Build history of the part. All positions in model axes, mm. A direction names the side the tool comes from. Give positions to 0.01 mm unless a question says otherwise; leave off trailing zeros. Order: outer loops, then holes, each group sorted by start corner. A loop starts at its lowest first (then second) coordinate and runs counter-clockwise, first axis right, second up. Notation, with made-up numbers: (22.25, 9.5) - (29.25, 9.5) arc R6 cw to (29.25, 14.5) - close; hole circle Ø3 at (84.25, -36). An arc over 180 degrees is marked (long way). Use a Markdown table: item, result.
from build123d import *

# Parameters (mm, degrees)
SKETCH_1_R      = 1.5
SKETCH_1_R_2    = 15
EXTRUDE_1_DEPTH = 1.5


with BuildPart() as part:
    # 草圖1 → 填料-伸長1 (new body)
    with BuildSketch(Plane(origin=(0, 0, 0), x_dir=(1, 0, 0), z_dir=(0, 1, 0))):
        with BuildLine():
            Line((0, -3.980931511), (12.319060855, 2.328849967))
            ThreePointArc((12.319060855, 2.328849967), (14.431141465, 4.388450613), (15.014493405, 7.28025625))
            ThreePointArc((15.014493405, 7.28025625), (11.971039141, 65.394509034), (14.52184689, 123.53246884))
            ThreePointArc((14.52184689, 123.53246884), (15.377876917, 128.098069479), (17.067022361, 132.425226083))
            ThreePointArc((17.067022361, 132.425226083), (16.965589985, 149.77375384), (2.866920195, 159.883611111))
            ThreePointArc((2.866920195, 159.883611111), (0, 162), (-2.866920195, 159.883611111))
            ThreePointArc((-2.866920195, 159.883611111), (-16.965589985, 149.77375384), (-17.067022361, 132.425226083))
            ThreePointArc((-17.067022361, 132.425226083), (-15.377876917, 128.098069479), (-14.52184689, 123.53246884))
            ThreePointArc((-14.52184689, 123.53246884), (-11.971039141, 65.394509034), (-15.014493405, 7.28025625))
            ThreePointArc((-15.014493405, 7.28025625), (-14.431141465, 4.388450613), (-12.319060855, 2.328849967))
            Line((-12.319060855, 2.328849967), (0, -3.980931511))
        make_face()
        with Locations(Location((-12, 127.583592135, 0), (0, 0, 270))):
            Circle(SKETCH_1_R, mode=Mode.SUBTRACT)
        with Locations(Location((12, 127.583592135, 0), (0, 0, 270))):
            Circle(SKETCH_1_R, mode=Mode.SUBTRACT)
        with Locations(Location((8.6, 68.325395665, 0), (0, 0, 270))):
            Circle(SKETCH_1_R, mode=Mode.SUBTRACT)
        with Locations(Location((-8.6, 68.325395665, 0), (0, 0, 270))):
            Circle(SKETCH_1_R, mode=Mode.SUBTRACT)
        with Locations(Location((10.05, 6, 0), (0, 0, 270))):
            Circle(SKETCH_1_R, mode=Mode.SUBTRACT)
        with Locations(Location((-10.05, 6, 0), (0, 0, 270))):
            Circle(SKETCH_1_R, mode=Mode.SUBTRACT)
        with Locations(Location((0, 159, 0), (0, 0, 270))):
            Circle(SKETCH_1_R, mode=Mode.SUBTRACT)
        with Locations(Location((0, 0, 0), (0, 0, 270))):
            Circle(SKETCH_1_R, mode=Mode.SUBTRACT)
        with Locations(Location((0, 141, 0), (0, 0, 270))):
            Circle(SKETCH_1_R_2, mode=Mode.SUBTRACT)
        Polygon((0, 14.042409585), (-4.491071946, 11.449487988), (-5.101164168, 5.002829556), (5.101164168, 5.002829556), (4.491071946, 11.449487988), align=None, mode=Mode.SUBTRACT)
        with BuildLine():
            Line((0, 112.532142135), (-6.334048162, 108.875177723))
            ThreePointArc((-6.334048162, 108.875177723), (-6.614696141, 112.870067669), (-6.92146425, 116.863036776))
            Line((-6.92146425, 116.863036776), (-0.136378432, 120.780407899))
            ThreePointArc((-0.136378432, 120.780407899), (0, 120.816950389), (0.136378432, 120.780407899))
            Line((0.136378432, 120.780407899), (6.92146425, 116.863036776))
            ThreePointArc((6.92146425, 116.863036776), (6.614696141, 112.870067669), (6.334048162, 108.875177723))
            Line((6.334048162, 108.875177723), (0, 112.532142135))
        make_face(mode=Mode.SUBTRACT)
        with BuildLine():
            Line((0, 102.344922167), (5.753985291, 99.02285721))
            ThreePointArc((5.753985291, 99.02285721), (5.547257407, 94.643430297), (5.371890331, 90.262635518))
            Line((5.371890331, 90.262635518), (0, 93.364097846))
            Line((0, 93.364097846), (-5.371890331, 90.262635518))
            ThreePointArc((-5.371890331, 90.262635518), (-5.547257407, 94.643430297), (-5.753985291, 99.02285721))
            Line((-5.753985291, 99.02285721), (0, 102.344922167))
        make_face(mode=Mode.SUBTRACT)
        with BuildLine():
            Line((0, 84.072725452), (5.10712289, 81.124126676))
            ThreePointArc((5.10712289, 81.124126676), (5.026699976, 76.609736924), (4.97956534, 72.094876904))
            Line((4.97956534, 72.094876904), (0, 74.969830293))
            Line((0, 74.969830293), (-4.97956534, 72.094876904))
            ThreePointArc((-4.97956534, 72.094876904), (-5.026699976, 76.609736924), (-5.10712289, 81.124126676))
            Line((-5.10712289, 81.124126676), (0, 84.072725452))
        make_face(mode=Mode.SUBTRACT)
        with BuildLine():
            Line((0, 65.619773758), (4.987851065, 62.740036603))
            ThreePointArc((4.987851065, 62.740036603), (5.046332025, 58.016878131), (5.141244155, 53.29431128))
            Line((5.141244155, 53.29431128), (0, 56.262609977))
            Line((0, 56.262609977), (-5.141244155, 53.29431128))
            ThreePointArc((-5.141244155, 53.29431128), (-5.046332025, 58.016878131), (-4.987851065, 62.740036603))
            Line((-4.987851065, 62.740036603), (0, 65.619773758))
        make_face(mode=Mode.SUBTRACT)
        with BuildLine():
            Line((0, 46.827706802), (5.447027498, 43.68286401))
            ThreePointArc((5.447027498, 43.68286401), (5.648052955, 39.057684109), (5.884040018, 34.434156186))
            Line((5.884040018, 34.434156186), (0, 37.831308275))
            Line((0, 37.831308275), (-5.884040018, 34.434156186))
            ThreePointArc((-5.884040018, 34.434156186), (-5.648052955, 39.057684109), (-5.447027498, 43.68286401))
            Line((-5.447027498, 43.68286401), (0, 46.827706802))
        make_face(mode=Mode.SUBTRACT)
        with BuildLine():
            Line((0, 28.460830008), (6.494782795, 24.711065414))
            ThreePointArc((6.494782795, 24.711065414), (6.852315766, 19.927479382), (7.247310233, 15.146840877))
            Line((7.247310233, 15.146840877), (0, 19.331077391))
            Line((0, 19.331077391), (-7.247310233, 15.146840877))
            ThreePointArc((-7.247310233, 15.146840877), (-6.852315766, 19.927479382), (-6.494782795, 24.711065414))
            Line((-6.494782795, 24.711065414), (0, 28.460830008))
        make_face(mode=Mode.SUBTRACT)
    extrude(amount=EXTRUDE_1_DEPTH)


solid = part.part
1) Slice it at D-D (z = 0). Write the cut outline in (x, y).
Computed:
| item | result |
|---|---|
| outline | (-7.77, 0) - (-1.5, 0) - (-1.5, 1.5) - (-7.77, 1.5) - close; (1.5, 0) - (7.77, 0) - (7.77, 1.5) - (1.5, 1.5) - close |
2) Slice it at A-A (z = -141). Write the cut outline in (x, y).
Computed:
| item | result |
|---|---|
| outline | (-19.1, 0) - (-15, 0) - (-15, 1.5) - (-19.1, 1.5) - close; (15, 0) - (19.1, 0) - (19.1, 1.5) - (15, 1.5) - close |
3) Slice it at B-B (z = -110.5). Write the cut outline in (x, y), and give its area (3 significant figures).
Computed:
| item | result |
|---|---|
| outline | (-13.46, 0) - (-6.45, 0) - (-6.45, 1.5) - (-13.46, 1.5) - close; (-3.52, 0) - (3.52, 0) - (3.52, 1.5) - (-3.52, 1.5) - close; (6.45, 0) - (13.46, 0) - (13.46, 1.5) - (6.45, 1.5) - close |
| area | 31.6 mm² |
4) Wall check: line 1 (X direction, y = 0.95, z = -62.5); line 2 (X direction, y = 0.9, z = -92.5); line 3 (Z direction, x = -9, y = 0.75). Give the ranges that are in metal, low to high. Write a range as from..to.
Computed:
| item | result |
|---|---|
| line 1 | x = -11.99..-4.99, 4.99..11.99 |
| line 2 | x = -12.46..-5.46, -1.5..1.5, 5.46..12.46 |
| line 3 | z = -157.85..-153, -129..-69.77, -66.88..-7.07, -4.93..-0.63 |
5) Tool access for faces 1 (the flat face through (-6.25, 0.74, 0.78)), 2 (the flat face through (2.724, 0.74, -91.792)): list every direction of +Z, -Z, +X, -X, +Y, -Y with a clear straight run to the whole face (end or side of a thin tool).
Computed:
| item | result |
|---|---|
| face 1 | +Z, -X, +Y, -Y |
| face 2 | +Y, -Y |
6) Slice it at C-C (y = 0.9). State how many separate pieces and enclosed holes the cut face has, and give its area (3 significant figures).
Computed:
| item | result |
|---|---|
| separate pieces | 1 |
| enclosed holes | 16 |
| area | 2,930 mm² |
